Work out the finished part from the listing and answer in its coordinate system (mm). A direction names the side the tool comes from. Round coordinates to 2 decimals unless told otherwise and drop trailing zeros. Order: outer loops, then holes, each group sorted by start corner. A loop starts at its lowest first (then second) coordinate and runs counter-clockwise, first axis right, second up. Notation, with made-up numbers: (4.25, 20) - (13.25, 20) arc R12 cw to (13.25, 31) - close; hole circle Ø7 at (-38.75, -1). An arc over 180 degrees is marked (long way). Use CSV: the item, a comma, the result in double quotes.
from build123d import *

# Parameters (mm, degrees)
F1_DEPTH = 60
F2_R     = 41.0093140969
F3_DEPTH = 25


with BuildPart() as f1:
    # F0 (on Top) → F1 (new body)
    with BuildSketch(Plane.XY):
        Polygon((111.0508568783, 217.1731047251), (53.9866397324, 177.8834735035), (59.4803499027, 108.8195961973), (122.0382772188, 79.0453501127), (179.1024943647, 118.3349813343), (173.6087841944, 187.3988586405), align=None)
    extrude(amount=F1_DEPTH)

    # F2 (on face) → F3 (join)
    with BuildSketch(Plane.XY.offset(60)):
        with Locations((113.3089438081, 153.4131914377)):
            Circle(F2_R)
    extrude(amount=F3_DEPTH)


solid = f1.part
(1) Find section C-C (z = 51.5). Determine the outline of the cut face in (x, y).
Findings below:
outline,"(53.99, 177.88) - (59.48, 108.82) - (122.04, 79.05) - (179.1, 118.33) - (173.61, 187.4) - (111.05, 217.17) - close"
(2) Each of these flat-tipped pins is pushed along its axis until it touches: pin 1 (1.5 mm diameter, centred on y = 133, z = 30, fed in from +X); pin 2 (12 mm diameter, centred on y = 185.5, z = 44, fed in from +X); pin 3 (5 mm diameter, centred on x = 83, z = 30, fed in from -Y). Where does it stop, or does it pass through?
Findings below:
pin 1,"stops at x = 178"
pin 2,"stops at x = 174.24"
pin 3,"stops at y = 96.44"
(3) Find the intervals of material crossed by L1, parallel to Z at x = 158.5, y = 148; L2, parallel to Y at x = 165, z = 18.5; L3, parallel to Y at x = 130, z = 9, in increasing order. Write a range as from..to.
Findings below:
L1,"z = 0..60"
L2,"y = 108.63..191.5"
L3,"y = 84.53..208.15"
(4) Find section D-D (x = 160.5). Determine the outline of the cut face in (y, z), and give its area (3 significant figures).
Findings below:
outline,"(105.53, 0) - (193.64, 0) - (193.64, 60) - (105.53, 60) - close"
area,"5,290 mm²"
(5) Find section B-B (x = 105.5). Determine the outline of the cut face in (y, z).
Findings below:
outline,"(86.92, 0) - (213.35, 0) - (213.35, 60) - (193.67, 60) - (193.67, 85) - (113.15, 85) - (113.15, 60) - (86.92, 60) - close"
(6) For faces 1 (the cylindrical face through (80.765, 128.46, 72.325)), 2 (the flat face through (82.918, 197.803, 29.58)), determine the directions among +Z, -Z, +X, -X, +Y, -Y from which every point of the face is accessible in a straight line to the end or side of a thin tool.
Findings below:
face 1,"+Z"
face 2,"+Z, -Z, -X, +Y"
(7) Find section A-A (y = 164). Determine the outline of the cut face in (x, z).
Findings below:
outline,"(55.09, 0) - (175.47, 0) - (175.47, 60) - (152.93, 60) - (152.93, 85) - (73.69, 85) - (73.69, 60) - (55.09, 60) - close"
